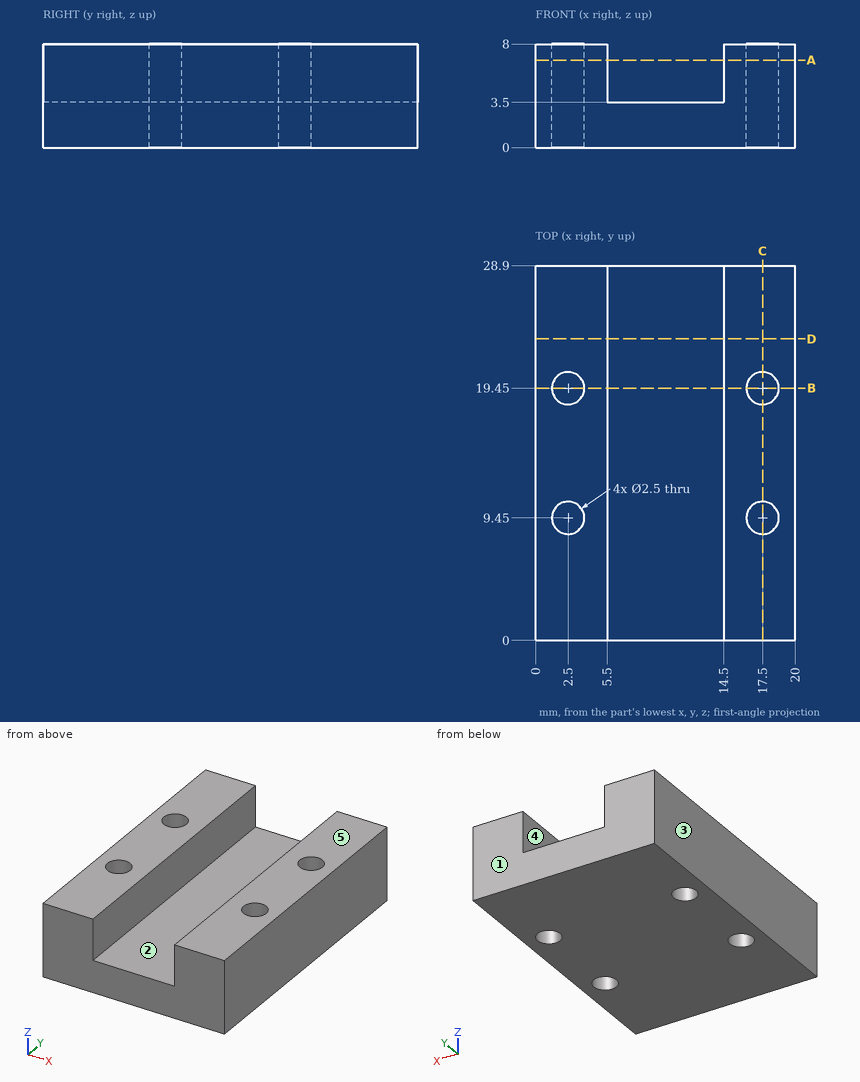
Job drawing, mm, ordinate dimensions from the low corner. One solid piece. A direction names the side the tool comes from. Round coordinates to 2 decimals unless told otherwise and drop trailing zeros. Loops run counter-clockwise (first coordinate to the right, second up) from the corner with the lowest first, then second, coordinate; pieces in that order, holes last.
(1) Cut at A-A (z = 6.75). Give the cut face in (x, y).
(2) Cut at B-B (y = 19.45). Give the cut face in (x, z).
(3) Drop flat-ended pins along their axis: pin 1 (2 mm diameter, centred on x = 9, z = 6, fed in from -Y); pin 2 (6 mm diameter, centred on x = 10, y = 24, fed in from +Z). Give the stop position or say it passes through.
(4) Wall check: line 1 along Y through (x, z) = (2.5, 3.5); line 2 along X through (y, z) = (16, 7); line 3 along X through (y, z) = (18.5, 2). Give the ranges that are in metal, low to high.
(5) Cut at D-D (y = 23.25). Give the cut face in (x, z).
(6) Two-plate mould, pull along X, no slides. Class the marked faces 3, 4 and 5: +X half, -X half, draft (parallel to the pull), parting line (faces both ways), or undercut.
(7) Cut at C-C (x = 17.5). Give the cut face in (y, z), plus the area to 3 significant figures.
(8) Which spindle directions (+Z, -Z, +X, -X, +Y, -Y) get a long thin tool onto all of the face, cutting with end or side? Do the marked faces 1 and 2. Say none if no direction does.
Findings below:
1. outline: (0, 0) - (5.5, 0) - (5.5, 28.9) - (0, 28.9) - close; (14.5, 0) - (20, 0) - (20, 28.9) - (14.5, 28.9) - close; hole circle Ø2.5 at (2.5, 9.45); hole circle Ø2.5 at (2.5, 19.45); hole circle Ø2.5 at (17.5, 9.45); hole circle Ø2.5 at (17.5, 19.45)
2. outline: (0, 0) - (1.25, 0) - (1.25, 8) - (0, 8) - close; (3.75, 0) - (16.25, 0) - (16.25, 8) - (14.5, 8) - (14.5, 3.5) - (5.5, 3.5) - (5.5, 8) - (3.75, 8) - close; (18.75, 0) - (20, 0) - (20, 8) - (18.75, 8) - close
3. pin 1: passes through
3. pin 2: stops at z = 3.5
4. line 1: y = 0 to 8.2, 10.7 to 18.2, 20.7 to 28.9
4. line 2: x = 0 to 5.5, 14.5 to 20
4. line 3: x = 0 to 1.69, 3.31 to 16.69, 18.31 to 20
5. outline: (0, 0) - (20, 0) - (20, 8) - (14.5, 8) - (14.5, 3.5) - (5.5, 3.5) - (5.5, 8) - (0, 8) - close
6. face 3: -X half
6. face 4: undercut
6. face 5: draft
7. outline: (0, 0) - (8.2, 0) - (8.2, 8) - (0, 8) - close; (10.7, 0) - (18.2, 0) - (18.2, 8) - (10.7, 8) - close; (20.7, 0) - (28.9, 0) - (28.9, 8) - (20.7, 8) - close
7. area: 191 mm2
8. face 1: +Z, -Z, +X, -X, +Y
8. face 2: +Z, +Y, -Y
